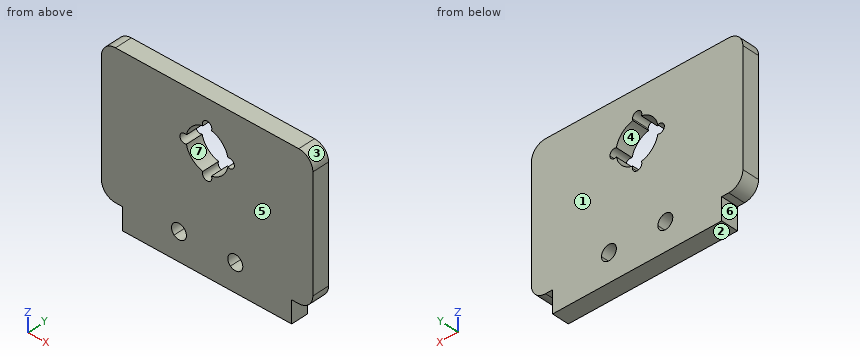
```python
from build123d import *

# Parameters (mm, degrees)
EXTRUDE_1_DEPTH     = 6
SKETCH_2_W          = 60
SKETCH_2_H          = 2
CUT_EXTRUDE_1_DEPTH = 10


with BuildPart() as part:
    # 草图1 → 凸台-拉伸1 (new body)
    with BuildSketch(Plane(origin=(0, 0, 0), x_dir=(1, 0, 0), z_dir=(0, 1, 0))):
        with BuildLine():
            ThreePointArc((-32.5, 33), (-36.035533906, 31.535533906), (-37.5, 28))
            Line((-37.5, 28), (-37.5, 13))
            Line((-37.5, 13), (-37.5, -12))
            ThreePointArc((-37.5, -12), (-36.035533906, -15.535533906), (-32.5, -17))
            Line((-32.5, -17), (32.5, -17))
            ThreePointArc((32.5, -17), (36.035533906, -15.535533906), (37.5, -12))
            Line((37.5, -12), (37.5, 13))
            Line((37.5, 13), (37.5, 28))
            ThreePointArc((37.5, 28), (36.035533906, 31.535533906), (32.5, 33))
            Line((32.5, 33), (30, 33))
            Line((30, 33), (30, 42.800232859))
            Line((30, 42.800232859), (-30, 42.800232859))
            Line((-30, 42.800232859), (-30, 33))
            Line((-30, 33), (-32.5, 33))
        make_face()
        with BuildLine():
            ThreePointArc((1.514624984, 7.34546875), (5.303300859, 5.303300859), (7.34546875, 1.514624984))
            ThreePointArc((7.34546875, 1.514624984), (8.906234914, 1.378853974), (9.65, 0))
            ThreePointArc((9.65, 0), (8.906234914, -1.378853974), (7.34546875, -1.514624984))
            ThreePointArc((7.34546875, -1.514624984), (5.303300859, -5.303300859), (1.514624984, -7.34546875))
            ThreePointArc((1.514624984, -7.34546875), (1.615801848, -7.665807858), (1.65, -8))
            ThreePointArc((1.65, -8), (-0.334192142, -9.615801848), (-1.514624984, -7.34546875))
            ThreePointArc((-1.514624984, -7.34546875), (-5.303300859, -5.303300859), (-7.34546875, -1.514624984))
            ThreePointArc((-7.34546875, -1.514624984), (-9.65, 0), (-7.34546875, 1.514624984))
            ThreePointArc((-7.34546875, 1.514624984), (-5.303300859, 5.303300859), (-1.514624984, 7.34546875))
            ThreePointArc((-1.514624984, 7.34546875), (-0.334192142, 9.615801848), (1.65, 8))
            ThreePointArc((1.65, 8), (1.615801848, 7.665807858), (1.514624984, 7.34546875))
        make_face(mode=Mode.SUBTRACT)
        with BuildLine():
            ThreePointArc((-7.35, 31), (-11.098950694, 28.588608831), (-11.738533865, 33))
            ThreePointArc((-11.738533865, 33), (-10, 33.65), (-8.261466135, 33))
            ThreePointArc((-8.261466135, 33), (-7.588608831, 32.098950694), (-7.35, 31))
        make_face(mode=Mode.SUBTRACT)
        with BuildLine():
            ThreePointArc((12.65, 31), (8.901049306, 28.588608831), (8.261466135, 33))
            ThreePointArc((8.261466135, 33), (10, 33.65), (11.738533865, 33))
            ThreePointArc((11.738533865, 33), (12.411391169, 32.098950694), (12.65, 31))
        make_face(mode=Mode.SUBTRACT)
    extrude(amount=EXTRUDE_1_DEPTH)

    # 草图2 → 切除-拉伸1 (cut)
    with BuildSketch(Plane(origin=(0, 6, 0), x_dir=(1, 0, 0), z_dir=(0, 1, 0))):
        with Locations((0, 41.800232859)):
            Rectangle(SKETCH_2_W, SKETCH_2_H)
    extrude(amount=-CUT_EXTRUDE_1_DEPTH, mode=Mode.SUBTRACT)


solid = part.part
```
Input: part model. Units: mm. Frame: model coordinates. Face numbers are marked on the shaded views. A direction names the side the tool comes from. Give positions to 0.01 mm unless a question says otherwise; leave off trailing zeros. Loops run counter-clockwise (first coordinate to the right, second up) from the corner with the lowest first, then second, coordinate; pieces in that order, holes last. Notation, with made-up numbers: (16.5, -38.5) -> (48.5, -38.5) arc R19 ccw to (48.5, -15.5) -> close; hole circle Ø3 at (19.5, 61). An arc over 180 degrees is marked (long way). Use a Markdown table: item, result.
Q1. Section query A-A, the plane x = 0. Return the cut outline in (y, z), plus the area to 3 significant figures.
Entries:
| item | result |
|---|---|
| outline | (0, -40.8) -> (6, -40.8) -> (6, -9.65) -> (0, -9.65) -> close; (0, 9.65) -> (6, 9.65) -> (6, 17) -> (0, 17) -> close |
| area | 231 mm² |
Q2. Access query for the marked faces 5, 6 and 7. Directions: +Z, -Z, +X, -X, +Y, -Y. A direction counts if a zero-diameter tool reaches every point of the face in a straight line with its end or side. Return the directions, or none.
Entries:
| item | result |
|---|---|
| face 5 | +Z, -Z, +X, -X, -Y |
| face 6 | -Z, -X, +Y, -Y |
| face 7 | +Y, -Y |
Q3. Section query C-C, the plane z = -5. Return the cut outline in (x, y).
Entries:
| item | result |
|---|---|
| outline | (-37.5, 0) -> (-5.59, 0) -> (-5.59, 6) -> (-37.5, 6) -> close; (5.59, 0) -> (37.5, 0) -> (37.5, 6) -> (5.59, 6) -> close |
Q4. First-contact query: P1, Ø2, axis at x = -31.5, y = 3, coming from the -Z side; P2, Ø1.8, axis at y = 2.5, z = -38, coming from the +X side. Flat tips, straight axial feed; report the tip coordinate or a pass-through.
Entries:
| item | result |
|---|---|
| P1 | stops at z = -33 |
| P2 | stops at x = 30 |
Q5. Pull-direction query (Z, two-part tool) for the marked faces 1, 2, 3 and 4; classes: pulls with the +Z half, pulls with the -Z half, needs draft (parallel to the pull), parting line crosses it, or undercut.
Entries:
| item | result |
|---|---|
| face 1 | needs draft |
| face 2 | pulls with the -Z half |
| face 3 | pulls with the +Z half |
| face 4 | undercut |
Q6. Section query B-B, the plane y = 5.1. Return the cut outline in (x, z).
Entries:
| item | result |
|---|---|
| outline | (-37.5, -28) arc R5 ccw to (-32.5, -33) -> (-30, -33) -> (-30, -40.8) -> (30, -40.8) -> (30, -33) -> (32.5, -33) arc R5 ccw to (37.5, -28) -> (37.5, 12) arc R5 ccw to (32.5, 17) -> (-32.5, 17) arc R5 ccw to (-37.5, 12) -> close; hole circle Ø5.3 at (-10, -31); hole (-7.35, -1.51) arc R7.5 ccw to (-1.51, -7.35) arc R1.65 ccw (long way) to (1.51, -7.35) arc R7.5 ccw to (7.35, -1.51) arc R1.65 ccw (long way) to (7.35, 1.51) arc R7.5 ccw to (1.51, 7.35) arc R1.65 ccw (long way) to (-1.51, 7.35) arc R7.5 ccw to (-7.35, 1.51) arc R1.65 ccw (long way) to start; hole circle Ø5.3 at (10, -31) |
Q7. Ray query, probe 1 along Z at (x, y) = (0, 2.6); probe 2 along Z at (x, y) = (-10, 3.9); probe 3 along X at (y, z) = (3.55, 8). Return the intervals inside material, ascending. Write a range as from..to.
Entries:
| item | result |
|---|---|
| probe 1 | z = -40.8..-9.65, 9.65..17 |
| probe 2 | z = -40.8..-33.65, -28.35..17 |
| probe 3 | x = -37.5..-1.65, 1.65..37.5 |
